Autodesk Inventor part; units mm, degrees
ref_plane "YZ Plane" through (0, 0, 0) normal (1, 0, 0) x (0, 1, 0)
ref_plane "XZ Plane" through (0, 0, 0) normal (0, 1, 0) x (-1, 0, 0)
ref_plane "XY Plane" through (0, 0, 0) normal (0, 0, 1) x (1, 0, 0)
sketch "Sketch1" plane through (0, 0, 0) normal (0, 0, 1) x (1, 0, 0)
  circle A0 centre (0.8326, 3.0356) radius 2.5
  point P0 (0, 0)
  dimension "d0" = 5
extrude "Extrusion1" add sketch "Sketch1" along normal blind 29.972
sketch "Sketch2" plane through (0.8326, 3.0356, 29.972) normal (0, 0, 1) x (1, 0, 0)
  circle A0 centre (0, 0) radius 2.5
  circle A1 centre (0, 0) radius 5.015
  point P0 (-0.8326, -3.0356)
extrude "Extrusion2" add sketch "Sketch2" along normal blind 7.5 contours A0 | A1
sketch "Sketch3" plane through (0.8326, 3.0356, 0) normal (0, 0, -1) x (-1, 0, 0)
  circle A0 centre (0, 0) radius 5.015
  circle A1 centre (0, 0) radius 2.5
  circle A2 centre (0, 0) radius 2.5
  point P0 (0.8326, -3.0356)
extrude "Extrusion3" add sketch "Sketch3" along normal blind 6 contours A1
properties part number "5mm_bolt" material "Steel, Alloy"
Geometry check sheet. Reference: the model listing, model coordinates, mm. A direction names the side the tool comes from. Give positions to 0.01 mm unless a question says otherwise; leave off trailing zeros. Write each loop counter-clockwise with the first axis right and the second up, starting at its lowest first coordinate (ties: lowest second). Pieces come first, ordered by that corner, then holes.
1) Section check A-A, the plane x = 2. Record the boundary of the cut face in (y, z), and give its area (3 significant figures).
2) Section check B-B, the plane y = 4. Record the boundary of the cut face in (x, z).
3) Material ranges on L1, parallel to X at y = 3, z = 14; L2, parallel to Z at x = 4.5, y = 4; L3, parallel to X at y = 6.5, z = 35.5, recorded low to high.
4) Access from +Z, -Z, +X, -X, +Y, -Y to the whole of each face (thin tool, end or side, straight path). Record for faces 1 (the flat face through (3, 1, 29.972)), 2 (the cylindrical face through (5.616, 1.529, 33.67)).
5) Section check D-D, the plane x = 4.25. Record the boundary of the cut face in (y, z).
6) Section check C-C, the plane z = 9.5. Record the boundary of the cut face in (x, y), and give its area (3 significant figures).
7) Gauge pin test, flat ends, axial feed: pin 1 (1.5 mm diameter, centred on x = -2.5, y = 0.5, fed in from -Z); pin 2 (1.5 mm diameter, centred on x = 3, z = 30.5, fed in from +Y); pin 3 (4 mm diameter, centred on x = 1, z = 1.5, fed in from -Y). Record the tip position at first contact, or that the pin passes through.
Computed:
1. outline: (-1.84, 29.97) - (0.82, 29.97) - (0.82, -6) - (5.25, -6) - (5.25, 29.97) - (7.91, 29.97) - (7.91, 37.47) - (-1.84, 37.47) - close
1. area: 232 mm2
2. outline: (-4.09, 29.97) - (-1.47, 29.97) - (-1.47, -6) - (3.14, -6) - (3.14, 29.97) - (5.75, 29.97) - (5.75, 37.47) - (-4.09, 37.47) - close
3. L1: x = -1.67 to 3.33
3. L2: z = 29.97 to 37.47
3. L3: x = -2.79 to 4.46
4. face 1: -Z
4. face 2: +Z, -Z
5. outline: (-0.63, 29.97) - (6.71, 29.97) - (6.71, 37.47) - (-0.63, 37.47) - close
6. outline: circle Ø5 at (0.83, 3.04)
6. area: 19.6 mm2
7. pin 1: stops at z = 29.97
7. pin 2: stops at y = 7.85
7. pin 3: stops at y = 0.54
